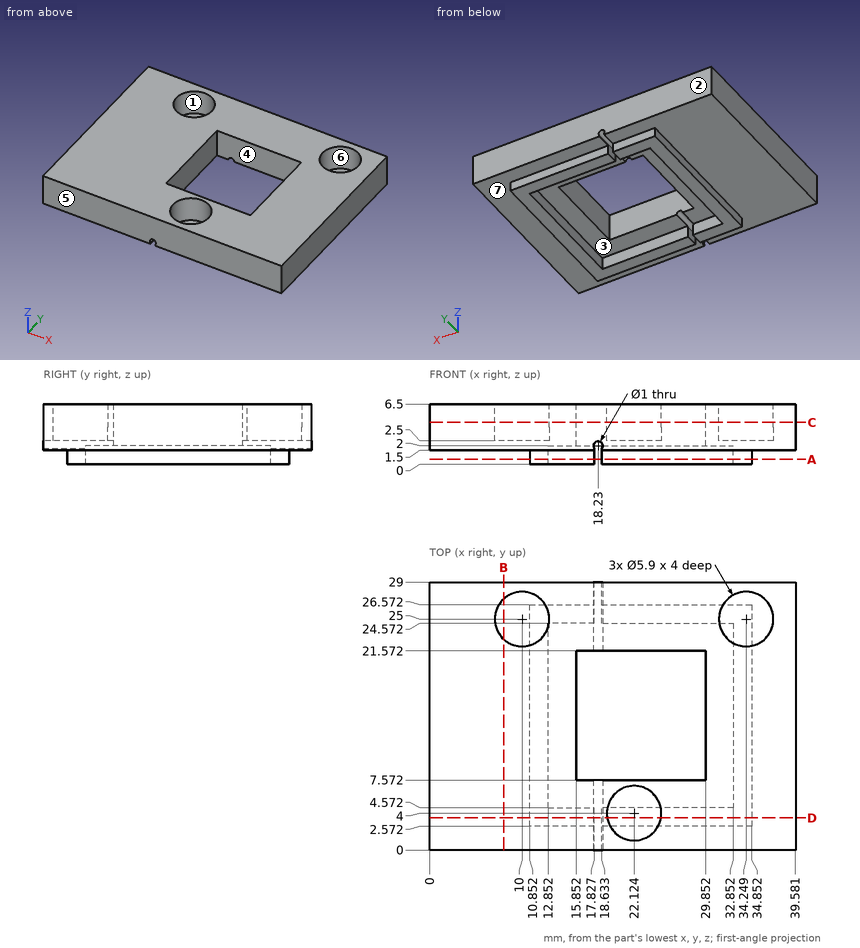
Can you work these out from the drawing? Everything is in mm from the part's minimum corner. A direction names the side the tool comes from. Give positions to 0.01 mm unless a question says otherwise; leave off trailing zeros. Loops run counter-clockwise (first coordinate to the right, second up) from the corner with the lowest first, then second, coordinate; pieces in that order, holes last. Notation, with made-up numbers: (-35, 32.25) - (12, 32.25) arc R14 ccw to (12, 38.25) - close; hole circle Ø5 at (4.25, -23.75). An arc over 180 degrees is marked (long way). Answer as a JSON object with one key per item and string values.
Q1. Which directions (+Z, -Z, +X, -X, +Y, -Y) give clear straight access to the entire face, cutting with the end or side of a thin tool? Please do the marked faces 1, 2, 3 and 4.
Geometry says:
{"face 1": "+Z", "face 2": "+Z, -Z, +X, -X, +Y", "face 3": "-Z", "face 4": "+Z, -Z"}
Q2. If I drill on L1, parallel to X at y = 25, z = 4.4; L2, parallel to Y at x = 27.5, z = 1.75; L3, parallel to Y at x = 13.5, z = 0.75, over which ranges is the centre line in solid material (lowest first)?
Geometry says:
{"L1": "0 to 7.05, 12.95 to 31.3, 37.2 to 39.58", "L2": "0 to 4.57, 24.57 to 29", "L3": "2.57 to 4.57, 24.57 to 26.57"}
Q3. Imagine slicing it at C-C on z = 4.5. Give the number of separate pieces and of enclosed holes in the cut face, plus the area to 3 significant figures.
Geometry says:
{"separate pieces": "1", "enclosed holes": "4", "area": "870 mm²"}
Q4. If we mould it in two halves opening along Y, with no side actions, what happens to the marked faces 5, 6 and 7? For each: pulls with the +Y half, pulls with the -Y half, needs draft (parallel to the pull), parting line crosses it, or undercut.
Geometry says:
{"face 5": "pulls with the -Y half", "face 6": "undercut", "face 7": "needs draft"}
Q5. Will these pins go through, and if not, where does the flat tip stop? P1, Ø3, axis at x = 26.5, y = 8.5, coming from the -Z side; P2, Ø2, axis at x = 21, z = 4.5, coming from the -Y side; P3, Ø0.5, axis at y = 26.5, z = 0.5, coming from the -X side.
Geometry says:
{"P1": "z = 2", "P2": "y = 0", "P3": "x = 10.85"}
Q6. Imagine slicing it at D-D on y = 3.5. Write out the boundary of the cut face in (x, z).
Geometry says:
{"outline": "(0, 1.5) - (10.85, 1.5) - (10.85, 0) - (17.83, 0) - (17.83, 1.7) arc R0.5 cw (long way) to (18.63, 1.7) - (18.63, 0) - (34.85, 0) - (34.85, 1.5) - (39.58, 1.5) - (39.58, 6.5) - (25.03, 6.5) - (25.03, 2.5) - (19.22, 2.5) - (19.22, 6.5) - (0, 6.5) - close"}
Q7. Imagine slicing it at B-B on x = 8. Write out the boundary of the cut face in (y, z), plus the area to 3 significant figures.
Geometry says:
{"outline": "(0, 1.5) - (29, 1.5) - (29, 6.5) - (27.17, 6.5) - (27.17, 2.5) - (22.83, 2.5) - (22.83, 6.5) - (0, 6.5) - close", "area": "128 mm²"}
Q8. Imagine slicing it at A-A on z = 0.5. Write out the boundary of the cut face in (x, y).
Geometry says:
{"outline": "(10.85, 2.57) - (17.83, 2.57) - (17.83, 4.57) - (12.85, 4.57) - (12.85, 24.57) - (17.83, 24.57) - (17.83, 26.57) - (10.85, 26.57) - close; (18.63, 2.57) - (34.85, 2.57) - (34.85, 26.57) - (18.63, 26.57) - (18.63, 24.57) - (32.85, 24.57) - (32.85, 4.57) - (18.63, 4.57) - close"}
